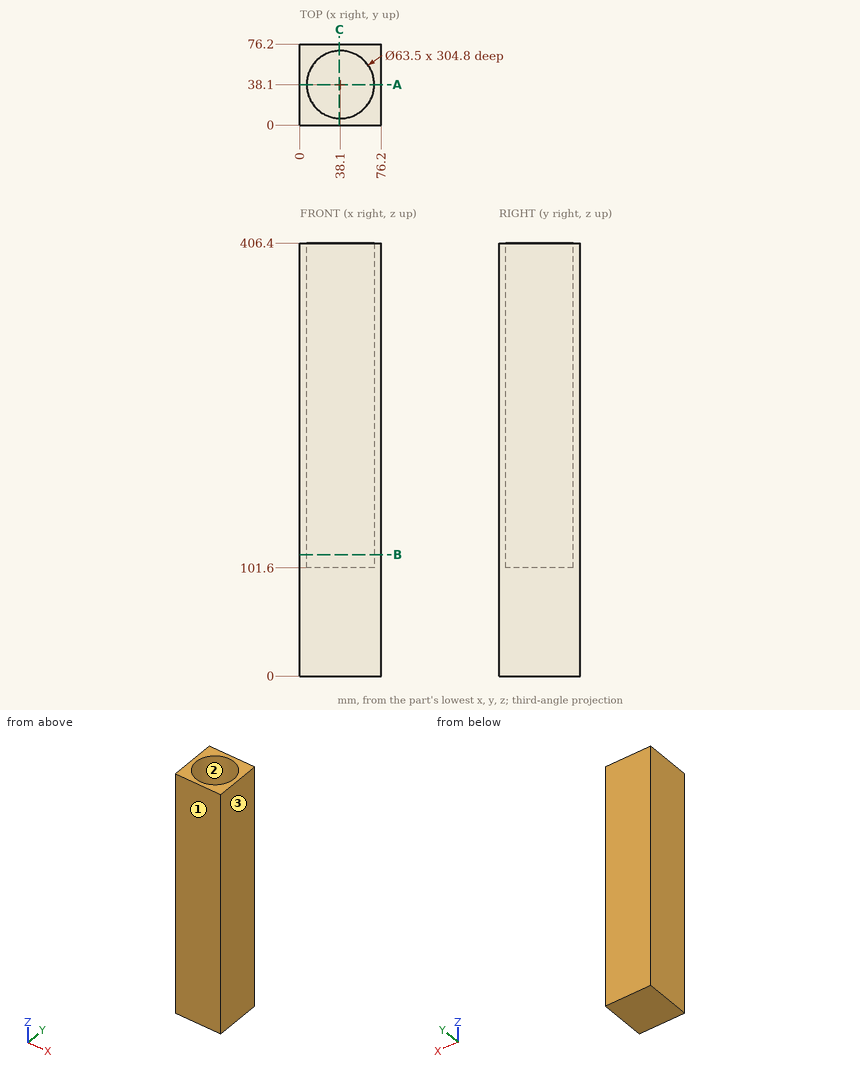
Could you check a few things on this drawing? It's one solid part, dimensions in mm from its lowest x, y, z. Coordinates: 2 decimals unless noted, no trailing zeros. Order: outer loops, then holes, each group sorted by start corner. A loop starts at its lowest first (then second) coordinate and runs counter-clockwise, first axis right, second up. Notation, with made-up numbers: M 88,62 L 122,62 A29 ccw 122,101 Z; hole C -2,89 d4. An arc over 180 degrees is marked long. Answer as a JSON object with one key per item and string values. Group by question number.
(1) I need wall thicknesses on probe 1 along Y at (x, z) = (39, 248.5); probe 2 along X at (y, z) = (38, 212); probe 3 along Z at (x, y) = (11.5, 21). Which ranges of each line are inside material? Lowest first, please.
(2) Suppose I cut it at C-C, the plane x = 37. Please give me the cut outline in (y, z), then the cut area to 3 significant figures.
(3) Suppose I cut it at B-B, the plane z = 114. Please give me the cut outline in (x, y), then the cut area to 3 significant figures.
(4) If we mould it in two halves opening along Y, with no side actions, what happens to the marked faces 1, 2 and 3? For each: released by +Y, released by -Y, zero draft, split by the parting line, or undercut.
(5) Suppose I cut it at A-A, the plane y = 38.1. Please give me the cut outline in (x, z).
(6) For pin 1 (6 mm diameter, centred on x = 53.5, y = 41, fed in from +Z), with a flat end and sliding along its axis, tell me the tip position at first contact or that it passes through.
Values found:
{
 "1": {"probe 1": "y = 0 to 6.36, 69.84 to 76.2", "probe 2": "x = 0 to 6.35, 69.85 to 76.2", "probe 3": "z = 0 to 101.6"},
 "2": {"outline": "M 0,0 L 76.2,0 L 76.2,406.4 L 69.83,406.4 L 69.83,101.6 L 6.37,101.6 L 6.37,406.4 L 0,406.4 Z", "area": "11,600 mm^2"},
 "3": {"outline": "M 0,0 L 76.2,0 L 76.2,76.2 L 0,76.2 Z; hole C 38.1,38.1 d63.5", "area": "2,640 mm^2"},
 "4": {"face 1": "released by -Y", "face 2": "undercut", "face 3": "zero draft"},
 "5": {"outline": "M 0,0 L 76.2,0 L 76.2,406.4 L 69.85,406.4 L 69.85,101.6 L 6.35,101.6 L 6.35,406.4 L 0,406.4 Z"},
 "6": {"pin 1": "stops at z = 101.6"}
}
